```python
from build123d import *

# Parameters (mm, degrees)
EXTRUDE_1_DEPTH     = 1
EXTRUDE_START       = 11.5
EXTRUDE_3_DEPTH     = 11.5
EXTRUDE_START_2     = 1
EXTRUDE_4_DEPTH     = 1
FILLET_1_R          = 1
FILLET_2_R          = 1
SKETCH_7_W          = 8.471052631578948
SKETCH_7_H          = 1
CUT_EXTRUDE_1_DEPTH = 1.5
SKETCH2_R           = 0.8000000000000002
CUT_EXTRUDE1_DEPTH  = 10


with BuildPart() as part:
    # 草图1 → 凸台-拉伸1 (new body)
    with BuildSketch(Plane(origin=(0, 0, 0), x_dir=(1, 0, 0), z_dir=(0, 1, 0))):
        with BuildLine():
            Line((13.595707880639235, -1.030263157894738), (10.075971038533972, -9.418398712579371))
            Line((10.075971038533972, -9.418398712579371), (7, -12.12435565298214))
            ThreePointArc((7, -12.12435565298214), (-12.93431345515802, 5.357568053111247), (13.522961568046952, 3.6234666314353032))
            Line((13.522961568046952, 3.6234666314353032), (13.595707880639235, -1.030263157894738))
        make_face()
        with BuildLine():
            Line((11.1, 0), (7.867624653739615, -7.830101040718992))
            ThreePointArc((7.867624653739615, -7.830101040718992), (-10.260132398183506, 4.235526315789474), (11.1, 0))
        make_face(mode=Mode.SUBTRACT)
    extrude(amount=EXTRUDE_1_DEPTH)

    # 草图2 → 凸台-拉伸3 (add)
    with BuildSketch(Plane(origin=(0, 0, 0), x_dir=(-1, 0, 0), z_dir=(0, -1, 0)).offset(EXTRUDE_START)):
        with BuildLine():
            Line((-13.595707880639234, -1.030263157894738), (-13.52296156804698, 3.6234666314351993))
            ThreePointArc((-13.52296156804698, 3.6234666314351993), (12.934313455157998, 5.357568053111296), (-7, -12.12435565298214))
            Line((-7, -12.12435565298214), (-10.07597103853397, -9.418398712579371))
            Line((-10.07597103853397, -9.418398712579371), (-13.595707880639234, -1.030263157894738))
        make_face()
        with BuildLine():
            Line((-9.226675534749763, -8.43317606696612), (-12.487400822321415, -0.5610888545377466))
            ThreePointArc((-12.487400822321415, -0.5610888545377466), (11.548494156391081, 4.783542904563626), (-9.226675534749763, -8.43317606696612))
        make_face(mode=Mode.SUBTRACT)
    extrude(amount=-EXTRUDE_3_DEPTH)

    # 草图5 → 凸台-拉伸4 (add)
    with BuildSketch(Plane(origin=(0, -11.5, 0), x_dir=(-1, 0, 0), z_dir=(0, -1, 0)).offset(EXTRUDE_START_2)):
        with BuildLine():
            Line((-13.522961568046979, 3.6234666314352), (-13.595707880639234, -1.030263157894738))
            Line((-13.595707880639234, -1.030263157894738), (-10.07597103853397, -9.418398712579371))
            Line((-10.07597103853397, -9.418398712579371), (-7.0000000000000115, -12.124355652982132))
            ThreePointArc((-7.0000000000000115, -12.124355652982132), (12.934313455157996, 5.3575680531112955), (-13.522961568046979, 3.6234666314352))
        make_face()
        with BuildLine():
            Line((-11.099999999999998, 0), (-7.867624653739613, -7.830101040718992))
            ThreePointArc((-7.867624653739613, -7.830101040718992), (10.260132398183506, 4.235526315789473), (-11.099999999999998, 0))
        make_face(mode=Mode.SUBTRACT)
    extrude(amount=-EXTRUDE_4_DEPTH)

    # 圆角1
    # the kernel refuses this fillet: 1 mm, written as the material it takes off along each edge
    with BuildSketch(Plane(origin=(11.953026446892592, -12.5, 7.767137681139568), x_dir=(-0.6605044125759219, 0, -0.7508221633434488), z_dir=(-0.7508221633434488, 0, 0.6605044125759219))) as fillet_1_piece_1:
        with BuildLine():
            CenterArc((FILLET_1_R, -FILLET_1_R), FILLET_1_R, 90, 90)
            Line((-1.17e-15, -FILLET_1_R), (0, 0))
            Line((0, 0), (FILLET_1_R, 0))
        make_face()
    extrude(amount=9.096803728910325, mode=Mode.SUBTRACT)
    with BuildSketch(Plane(origin=(1.33e-15, -12.5, -1.33e-15), x_dir=(0.6464264276811541, 0, 0.7629763257109501), z_dir=(0.7629763257109501, 0, -0.6464264276811541))) as fillet_1_piece_2:
        with BuildLine():
            CenterArc((14.000000000000002 - FILLET_1_R, -FILLET_1_R), FILLET_1_R, 0, 89.9999999999999)
            Line((14.000000000000002 - FILLET_1_R, 0), (14.000000000000002, 0))
            Line((14.000000000000002, 0), (14.000000000000002, -FILLET_1_R))
        make_face()
    revolve(axis=Axis((1.33e-15, -12.5, -1.33e-15), (0, -1, 0)), revolution_arc=305.54541710396313, mode=Mode.SUBTRACT)
    with BuildSketch(Plane(origin=(13.483886766982303, -12.5, -6.123161244767347), x_dir=(-1e-17, 1, 0), z_dir=(0.015629920425854232, 0, 0.9998778453328594))) as fillet_1_piece_3:
        with BuildLine():
            CenterArc((FILLET_1_R, FILLET_1_R), FILLET_1_R, 180, 90)
            Line((1e-17, FILLET_1_R), (0, 0))
            Line((0, 0), (FILLET_1_R, 0))
        make_face()
    extrude(amount=9.654298333593651, mode=Mode.SUBTRACT)
    with BuildSketch(Plane(origin=(14.563022756193803, -12.5, -1.275013817119511), x_dir=(9.6e-16, 1, 4e-16), z_dir=(-0.386925950221828, 0, 0.9221107900056997))) as fillet_1_piece_4:
        with BuildLine():
            CenterArc((FILLET_1_R, FILLET_1_R), FILLET_1_R, 180, 90.00000000000006)
            Line((-1.04e-15, FILLET_1_R), (0, 0))
            Line((0, 0), (FILLET_1_R, 0))
        make_face()
    extrude(amount=14.0966678251675, mode=Mode.SUBTRACT)

    # 圆角2
    # the kernel refuses this fillet: 1 mm, written as the material it takes off along each edge
    with BuildSketch(Plane(origin=(13.483886766982302, 1, -6.123161244767451), x_dir=(-1e-17, -1, 0), z_dir=(0.01562992042585999, 0, 0.9998778453328593))) as fillet_2_piece_1:
        with BuildLine():
            CenterArc((FILLET_2_R, -FILLET_2_R), FILLET_2_R, 90, 90)
            Line((1e-17, -FILLET_2_R), (0, 0))
            Line((0, 0), (FILLET_2_R, 0))
        make_face()
    extrude(amount=9.654298333593754, mode=Mode.SUBTRACT)
    with BuildSketch(Plane(origin=(-1.19e-15, 1, 1.55e-15), x_dir=(0.6464264276811535, 0, 0.7629763257109505), z_dir=(0.7629763257109505, 0, -0.6464264276811535))) as fillet_2_piece_2:
        with BuildLine():
            CenterArc((14.000000000000002 - FILLET_2_R, FILLET_2_R), FILLET_2_R, 270, 90)
            Line((14.000000000000002 - FILLET_2_R, 0), (14.000000000000002, 0))
            Line((14.000000000000002, 0), (14.000000000000002, FILLET_2_R))
        make_face()
    revolve(axis=Axis((-1.19e-15, 1, 1.55e-15), (0, -1, 0)), revolution_arc=305.54541710396273, mode=Mode.SUBTRACT)
    with BuildSketch(Plane(origin=(11.953026446892594, 1, 7.767137681139568), x_dir=(-0.6605044125759215, 0, -0.7508221633434492), z_dir=(-0.7508221633434492, 0, 0.6605044125759215))) as fillet_2_piece_3:
        with BuildLine():
            CenterArc((FILLET_2_R, FILLET_2_R), FILLET_2_R, 180, 90)
            Line((6.7e-16, FILLET_2_R), (0, 0))
            Line((0, 0), (FILLET_2_R, 0))
        make_face()
    extrude(amount=9.096803728910341, mode=Mode.SUBTRACT)
    with BuildSketch(Plane(origin=(14.563022756193805, 1, -1.2750138171195122), x_dir=(-0.9221107900056996, 0, -0.38692595022182796), z_dir=(-0.386925950221828, 0, 0.9221107900056997))) as fillet_2_piece_4:
        with BuildLine():
            CenterArc((FILLET_2_R, FILLET_2_R), FILLET_2_R, 180, 90)
            Line((-1e-17, FILLET_2_R), (0, 0))
            Line((0, 0), (FILLET_2_R, 0))
        make_face()
    extrude(amount=14.096667825167504, mode=Mode.SUBTRACT)

    # 草图7 → 切除-拉伸1 (cut)
    with BuildSketch(Plane(origin=(9.483812326869804, 0, 3.915050520359493), x_dir=(-0.3815789473684208, 0, 0.9243362520886044), z_dir=(-0.9243362520886044, 0, -0.3815789473684208))):
        with Locations((2.66e-15, 0.5)):
            Rectangle(SKETCH_7_W, SKETCH_7_H)
    extrude(amount=-CUT_EXTRUDE_1_DEPTH, mode=Mode.SUBTRACT)

    # Sketch2 → Cut-Extrude1 (cut)
    with BuildSketch(Plane(origin=(-13.134678702914778, 0, 4.845638799084908), x_dir=(0.3461170570774934, 0, 0.938191335922484), z_dir=(-0.938191335922484, 0, 0.34611705707749346))):
        with Locations((0, -5.75)):
            Circle(SKETCH2_R)
    extrude(amount=-CUT_EXTRUDE1_DEPTH, mode=Mode.SUBTRACT)


solid = part.part
```
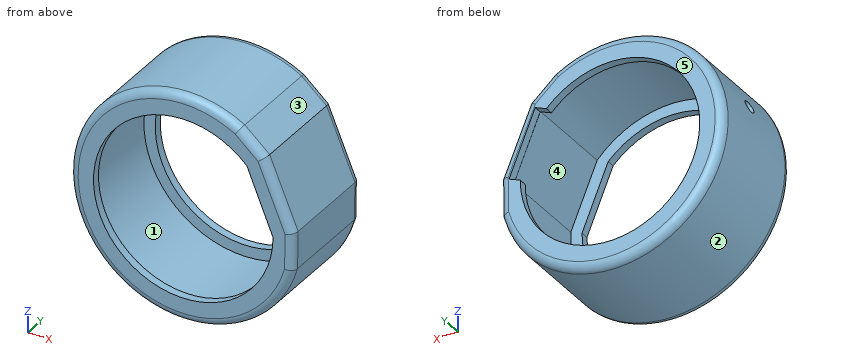
Work out the finished part from the listing and answer in its coordinate system (mm). Face numbers are marked on the shaded views. A direction names the side the tool comes from. Give positions to 0.01 mm unless a question says otherwise; leave off trailing zeros. Loops run counter-clockwise (first coordinate to the right, second up) from the corner with the lowest first, then second, coordinate; pieces in that order, holes last. Notation, with made-up numbers: (49.25, 9) -> (101.25, 9) arc R28 cw to (101.25, 37) -> close; hole circle Ø2 at (-12, 49). An arc over 180 degrees is marked (long way). Put each result on its own line as item: value. Start each with the question number.
Item 1: Which of the six approach directions +Z, -Z, +X, -X, +Y, -Y give full straight-line access (tool end or side, diameter ignored) to the marked faces 1 and 2?
Item 2: Each of these flat-tipped pins is pushed along its axis until it touches: P1, Ø1.5, axis at y = -3, z = -1, coming from the +X side; P2, Ø4, axis at y = -5, z = -7.5, coming from the -X side; P3, Ø1.5, axis at x = 7, z = 5, coming from the +Y side; P4, Ø5, axis at y = -8, z = -4, coming from the -X side. Where does it stop, or does it pass through?
Item 3: The mould has two halves that part along Z. Classify the marked faces 3, 4 and 5: released by +Z, released by -Z, zero draft, split by the parting line, or undercut.
Item 4: The part is cut by section A-A (x = 0). Give the vertices of the cut face in (y, z).
Item 5: Find the intervals of material crossed by L1, parallel to Z at x = 0, y = -3.75; L2, parallel to Y at x = 11, z = -4.75; L3, parallel to Z at x = 0, y = -11.8, in increasing order. Write a range as [from, to].
Item 6: The part is cut by section B-B (y = -9.75). Give the vertices of the cut face in (x, z), then the cut area to 3 significant figures.
Answers below:
1. face 1: none
1. face 2: +Y, -Y
2. P1: x = 13.58
2. P2: x = -12.87
2. P3: through
2. P4: x = -13.92
3. face 3: released by +Z
3. face 4: undercut
3. face 5: zero draft
4. outline: (-12.5, -13) arc R1 ccw to (-11.5, -14) -> (0, -14) arc R1 ccw to (1, -13) -> (1, -11.1) -> (0, -11.1) -> (0, -12.5) -> (-11.5, -12.5) -> (-11.5, -11.1) -> (-12.5, -11.1) -> close; (-12.5, 11.1) -> (-11.5, 11.1) -> (-11.5, 12.5) -> (0, 12.5) -> (0, 11.1) -> (1, 11.1) -> (1, 13) arc R1 ccw to (0, 14) -> (-11.5, 14) arc R1 ccw to (-12.5, 13) -> close
5. L1: [-14, -12.5], [12.5, 14]
5. L2: [-12.5, -11.5], [0, 1]
5. L3: [-13.95, -11.1], [11.1, 13.95]
6. outline: (7, 12.12) arc R14 ccw (long way) to (13.52, -3.62) -> (13.6, 1.03) -> (10.08, 9.42) -> close; hole (9.23, 8.43) arc R12.5 ccw (long way) to (12.49, 0.56) -> close
6. area: 119 mm2
